Geometry: see drawing. Coordinates: mm, zero at the bounding-box minimum. A direction names the side the tool comes from. Give positions to 0.01 mm unless a question says otherwise; leave off trailing zeros. Order: outer loops, then holes, each group sorted by start corner. A loop starts at its lowest first (then second) coordinate and runs counter-clockwise, first axis right, second up. Notation, with made-up numbers: M 79,25.5 L 88,25.5 A31 ccw 88,51.5 Z; hole C 84.25,31.25 d6. An arc over 180 degrees is marked long. Answer as a JSON object with one key per item and string values. Group by question number.
1. Pin query (flat end, axial travel): P1, Ø1.1, axis at x = 9.5, y = 16.5, coming from the -Z side; P2, Ø0.7, axis at x = 9, y = 16, coming from the +Z side; P3, Ø8, axis at x = 4.5, y = 15, coming from the -Z side. Return the tip coordinate at first contact, or that it passes through.
2. Set-up query: the marked faces 1 and 2. Return all of +Z, -Z, +X, -X, +Y, -Y with unobstructed straight access to the full face (end or side cutting, diameter ignored); none if empty.
3. Material intervals for L1, parallel to Y at x = 10.75, z = 6; L2, parallel to X at y = 16, z = 6.5; L3, parallel to X at y = 16.5, z = 7.25, sorted ascending. Write a range as [from, to].
4. Section query A-A (y = 14.25). Output: boundary loops of the cut face in (x, z).
5. Section query D-D (x = 10.34). Output: boundary loops of the cut face in (y, z).
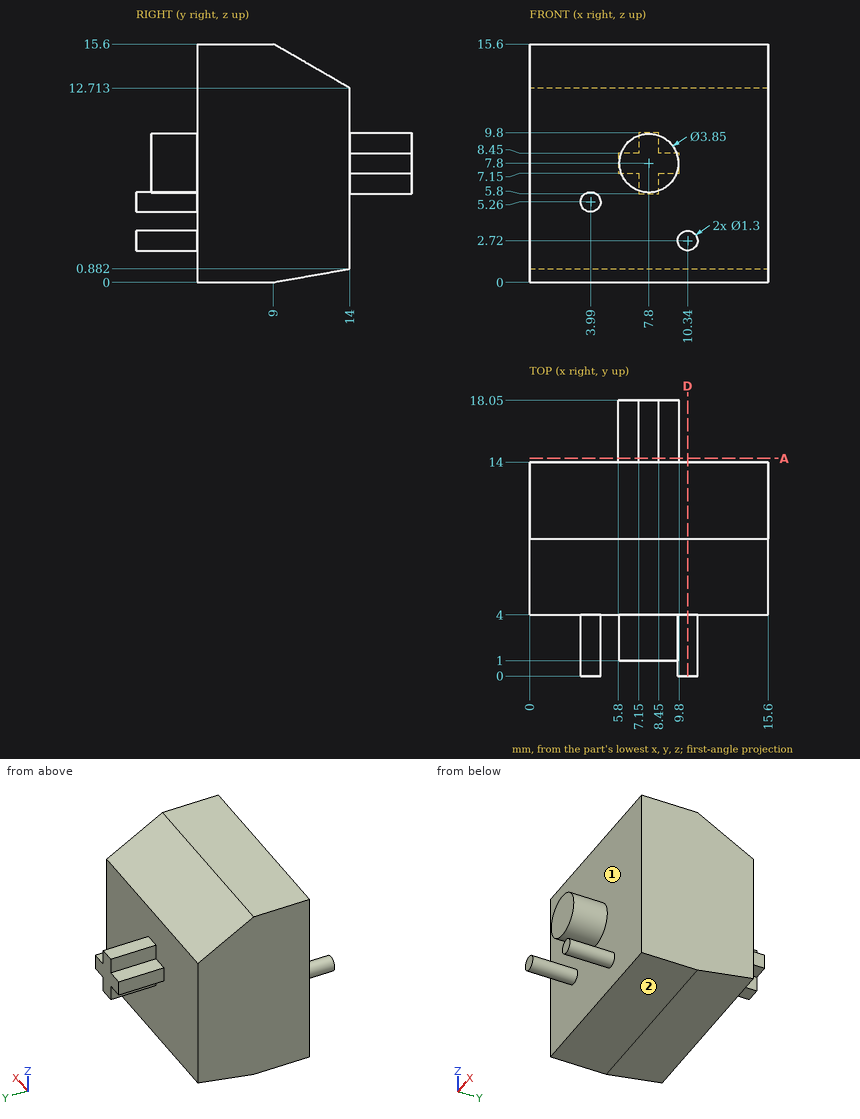
Answer sheet:
{
 "1": {"P1": "z = 7.15", "P2": "z = 8.45", "P3": "z = 0.35"},
 "2": {"face 1": "-Y", "face 2": "-Z, +X, -X, +Y, -Y"},
 "3": {"L1": "[4, 14]", "L2": "[7.15, 8.45]", "L3": "[5.8, 9.8]"},
 "4": {"outline": "M 5.8,7.15 L 7.15,7.15 L 7.15,5.8 L 8.45,5.8 L 8.45,7.15 L 9.8,7.15 L 9.8,8.45 L 8.45,8.45 L 8.45,9.8 L 7.15,9.8 L 7.15,8.45 L 5.8,8.45 Z"},
 "5": {"outline": "M 0,2.07 L 4,2.07 L 4,0 L 9,0 L 14,0.88 L 14,12.71 L 9,15.6 L 4,15.6 L 4,3.37 L 0,3.37 Z"}
}
